Input: part model. Units: mm. Frame: model coordinates. A direction names the side the tool comes from. Round coordinates to 2 decimals unless told otherwise and drop trailing zeros. Loops run counter-clockwise (first coordinate to the right, second up) from the corner with the lowest first, then second, coordinate; pieces in that order, holes last. Notation, with made-up numbers: (88, -0.75) - (94, -0.75) arc R31 ccw to (94, 25.25) - close; hole circle Ø9 at (14, 75.5). An arc over 180 degrees is marked (long way). One line per question, with ' | ' between items. Start each with the question number.
Item 1: Section C-C, the plane x = -25. Return loops of the section in (y, z) (3 decimals).
Item 2: Section A-A, the plane z = 5.75. Return loops of the section in (x, y), plus the area to 3 significant figures.
Item 3: Section B-B, the plane y = -11. Return loops of the section in (x, z) (3 decimals).
Item 4: Set-up query: faces 4 (the face through (-19.05, 1, 7)), 5 (the face through (-52, -19, 0)). Return all of +Z, -Z, +X, -X, +Y, -Y with unobstructed straight access to the full face (end or side cutting, diameter ignored); none if empty.
Item 5: Material intervals for line 1 along X through (y, z) = (2, 0.75); line 2 along Z through (x, y) = (-53.25, 0) (3 decimals); line 3 along Y through (x, z) = (-8, 3.75), sorted ascending.
Item 6: First-contact query: pin 1 (3 mm diameter, centred on x = -30.5, y = -19.5, fed in from +Z) (3 decimals). Flat tip, straight axial feed; report the tip coordinate or a pass-through.
Item 7: Draft query along X for faces 1 (the face through (0, -17, 2)), 2 (the face through (-52, -21, 3.175)), 3 (the face through (-62.23, 1, 7)). Return one class per face: pulls with the +X half, pulls with the -X half, needs draft (parallel to the pull), parting line crosses it, or undercut.
```python
from build123d import *

# Parameters (mm, degrees)
F0_W     = 101.6
F0_H     = 38.1
F1_DEPTH = 3.175
F3_DEPTH = 254
F2_R     = 3.81
F2_R_2   = 3.175
F4_DEPTH = 101.6
F5_START = -19.05
F5_DEPTH = 20.32
F6_START = -62.23
F6_DEPTH = 20.32


with BuildPart() as f1:
    # F0 (on Top) → F1 (new body)
    with BuildSketch(Plane.XY):
        with Locations((-50.8, -19.05)):
            Rectangle(F0_W, F0_H)
    extrude(amount=F1_DEPTH)

    # F2 (on face) → F3 (cut)
    with BuildSketch(Plane(origin=(-101.6, 0, 0), x_dir=(0, -1, 0), z_dir=(-1, 0, 0))):
        with BuildLine():
            ThreePointArc((3.7567106623, 3.175), (3.7966542918, 3.4913839483), (3.81, 3.81))
            ThreePointArc((3.81, 3.81), (-2.6940768363, 6.5040768363), (0, 0))
            Line((0, 0), (0, 0.635))
            ThreePointArc((0, 0.635), (-2.2450640303, 6.0550640303), (3.175, 3.81))
            ThreePointArc((3.175, 3.81), (3.1589222858, 3.4908840456), (3.1108519733, 3.175))
            Line((3.1108519733, 3.175), (3.7567106623, 3.175))
        make_face()
        with BuildLine():
            Line((0, 0.635), (0, 0))
            ThreePointArc((0, 0), (2.4593444248, 0.9000644337), (3.7567106623, 3.175))
            Line((3.7567106623, 3.175), (3.1108519733, 3.175))
            ThreePointArc((3.1108519733, 3.175), (2.0080463142, 1.3506555752), (0, 0.635))
        make_face()
        with BuildLine():
            Line((0, 3.175), (0, 0.635))
            ThreePointArc((0, 0.635), (2.0080463142, 1.3506555752), (3.1108519733, 3.175))
            Line((3.1108519733, 3.175), (0, 3.175))
        make_face()
    extrude(amount=-F3_DEPTH, mode=Mode.SUBTRACT)

    # F2 (on face) → F4 (join, through all)
    with BuildSketch(Plane(origin=(-101.6, 0, 0), x_dir=(0, -1, 0), z_dir=(-1, 0, 0))):
        with Locations((0, 3.81)):
            Circle(F2_R)
        with Locations((0, 3.81)):
            Circle(F2_R_2, mode=Mode.SUBTRACT)
    extrude(amount=-F4_DEPTH)

    # F2 (on face) → F5 (cut)
    with BuildSketch(Plane(origin=(-101.6, 0, 0), x_dir=(0, -1, 0), z_dir=(-1, 0, 0)).offset(F5_START)):
        with Locations((0, 3.81)):
            Circle(F2_R)
        with Locations((0, 3.81)):
            Circle(F2_R_2, mode=Mode.SUBTRACT)
    extrude(amount=-F5_DEPTH, mode=Mode.SUBTRACT)

    # F2 (on face) → F6 (cut)
    with BuildSketch(Plane(origin=(-101.6, 0, 0), x_dir=(0, -1, 0), z_dir=(-1, 0, 0)).offset(F6_START)):
        with Locations((0, 3.81)):
            Circle(F2_R)
        with Locations((0, 3.81)):
            Circle(F2_R_2, mode=Mode.SUBTRACT)
    extrude(amount=-F6_DEPTH, mode=Mode.SUBTRACT)


solid = f1.part
```
Return value:
1) outline: (-38.1, 0) - (0, 0) arc R3.81 cw to (-3.757, 3.175) - (-38.1, 3.175) - close
2) outline: (-101.6, -3.28) - (-82.55, -3.28) - (-82.55, -2.51) - (-101.6, -2.51) - close; (-101.6, 2.51) - (-82.55, 2.51) - (-82.55, 3.28) - (-101.6, 3.28) - close; (-62.23, -3.28) - (-39.37, -3.28) - (-39.37, -2.51) - (-62.23, -2.51) - close; (-62.23, 2.51) - (-39.37, 2.51) - (-39.37, 3.28) - (-62.23, 3.28) - close; (-19.05, -3.28) - (0, -3.28) - (0, -2.51) - (-19.05, -2.51) - close; (-19.05, 2.51) - (0, 2.51) - (0, 3.28) - (-19.05, 3.28) - close | area: 93.4 mm2
3) outline: (-101.6, 0) - (0, 0) - (0, 3.175) - (-101.6, 3.175) - close
4) face 4: +Z, +Y | face 5: -Z, +X, -X, +Y, -Y
5) line 1: -101.6 to -82.55, -62.23 to -39.37, -19.05 to 0 | line 2: 0 to 0.635, 6.985 to 7.62 | line 3: -3.81 to -3.17, 3.17 to 3.81
6) pin 1: z = 3.175
7) face 1: pulls with the +X half | face 2: needs draft | face 3: undercut
